from build123d import *

# Parameters (mm, degrees)
F0_W     = 48.9535877824
F0_H     = 15.875
F0_W_2   = 15.875
F0_H_2   = 65.8211410046
F0_W_3   = 122.4964122176
F0_H_3   = 69.2617977858
F1_DEPTH = 19.05


with BuildPart() as f1:
    # F0 (on Front) → F1 (new body)
    with BuildSketch(Plane.XZ):
        with Locations((-126.7005329192, 17.3074353337)):
            Rectangle(F0_W, F0_H)
        with Locations((-126.7005329192, 1.4324353337)):
            Rectangle(F0_W, F0_H)
        with Locations((-94.286239028, 1.4324353337)):
            Rectangle(F0_W_2, F0_H)
        with Locations((-94.286239028, -39.4156351686)):
            Rectangle(F0_W_2, F0_H_2)
        with Locations((-78.411239028, -39.4156351686)):
            Rectangle(F0_W_2, F0_H_2)
        with Locations((-78.411239028, 1.4324353337)):
            Rectangle(F0_W_2, F0_H)
        with Locations((-9.2255329192, 1.4324353337)):
            Rectangle(F0_W_3, F0_H)
        with Locations((-9.2255329192, 17.3074353337)):
            Rectangle(F0_W_3, F0_H)
        with Locations((-78.411239028, 17.3074353337)):
            Rectangle(F0_W_2, F0_H)
        with Locations((-94.286239028, 17.3074353337)):
            Rectangle(F0_W_2, F0_H)
        with Locations((-78.411239028, 59.8758342266)):
            Rectangle(F0_W_2, F0_H_3)
        with Locations((-94.286239028, 59.8758342266)):
            Rectangle(F0_W_2, F0_H_3)
    extrude(amount=F1_DEPTH)


solid = f1.part
Part model, mm, in its own coordinate system. A direction names the side the tool comes from. Give positions to 0.01 mm unless a question says otherwise; leave off trailing zeros. Order: outer loops, then holes, each group sorted by start corner. A loop starts at its lowest first (then second) coordinate and runs counter-clockwise, first axis right, second up. Notation, with made-up numbers: (66.25, 9) -> (115.25, 9) arc R17 ccw to (115.25, 42) -> close; hole circle Ø3 at (76, 43). An arc over 180 degrees is marked (long way). Use one line per item in the form item = value.
(1) Flat gauge pins, fed straight in: P1, Ø1.5, axis at y = -15.5, z = -39.5, coming from the +X side; P2, Ø6, axis at y = -8, z = -52.5, coming from the -X side; P3, Ø5, axis at x = 2, y = -10, coming from the +Z side. Where does each tip first touch, or does it go through?
Solution:
P1 = -70.47
P2 = -102.22
P3 = 25.24
(2) Saw through at C-C (x = 22.5). Write the cut outline in (y, z), then the cut area to 3 significant figures.
Solution:
outline = (-19.05, -6.51) -> (0, -6.51) -> (0, 25.24) -> (-19.05, 25.24) -> close
area = 605 mm²
(3) Saw through at A-A (y = -6.25). Write the cut outline in (x, z).
Solution:
outline = (-151.18, -6.51) -> (-102.22, -6.51) -> (-102.22, -72.33) -> (-70.47, -72.33) -> (-70.47, -6.51) -> (52.02, -6.51) -> (52.02, 25.24) -> (-70.47, 25.24) -> (-70.47, 94.51) -> (-102.22, 94.51) -> (-102.22, 25.24) -> (-151.18, 25.24) -> close
(4) Drill centre lines: line 1 (Z direction, x = 1, y = -14.5); line 2 (X direction, y = -8.5, z = 85). Where is each one in solid material? Low to high. Write a range as from..to.
Solution:
line_1 = -6.51..25.24
line_2 = -102.22..-70.47
(5) Saw through at B-B (z = 76). Write the cut outline in (x, y).
Solution:
outline = (-102.22, -19.05) -> (-70.47, -19.05) -> (-70.47, 0) -> (-102.22, 0) -> close
(6) Tool access for faces 1 (the face through (-102.224, -9, 59)), 2 (the face through (-70.474, -9, -40)), 3 (the face through (-102.224, -9, -40)), 4 (the face through (-87, -9, -72.326)), 5 (the face through (-8, -9, 25.245)): list every direction of +Z, -Z, +X, -X, +Y, -Y with a clear straight run to the whole face (end or side of a thin tool).
Solution:
face_1 = +Z, -X, +Y, -Y
face_2 = -Z, +X, +Y, -Y
face_3 = -Z, -X, +Y, -Y
face_4 = -Z, +X, -X, +Y, -Y
face_5 = +Z, +X, +Y, -Y
